Autodesk Inventor part; units mm, degrees
ref_plane "YZ Plane" through (0, 0, 0) normal (1, 0, 0) x (0, 1, 0)
ref_plane "XZ Plane" through (0, 0, 0) normal (0, 1, 0) x (-1, 0, 0)
ref_plane "XY Plane" through (0, 0, 0) normal (0, 0, 1) x (1, 0, 0)
sketch "スケッチ1" plane through (0, 0, 0) normal (0, 0, 1) x (1, 0, 0)
  circle A0 centre (0, 0) radius 1.5
  dimension "d0" = 3
extrude "押し出し1" add sketch "スケッチ1" along normal blind 15
sketch "スケッチ2" plane through (0, 0, 15) normal (0, 0, 1) x (1, 0, 0)
  circle A0 centre (0, 0) radius 1.5
  circle A1 centre (0, 0) radius 3
  dimension "d3" = 6
extrude "押し出し2" add sketch "スケッチ2" along normal blind 2 contours A0 | A1
fillet "フィレット1" radius 2 1 edges at (-3, 0, 17)
properties part number "M3ボタンボルト15" material "鋼、高強度、低合金"
Can you work these out from the model? Positions are in its coordinate system, mm. A direction names the side the tool comes from. Give positions to 0.01 mm unless a question says otherwise; leave off trailing zeros. Loops run counter-clockwise (first coordinate to the right, second up) from the corner with the lowest first, then second, coordinate; pieces in that order, holes last. Notation, with made-up numbers: (28, 62.25) -> (37, 62.25) arc R24 cw to (37, 94.25) -> close; hole circle Ø8 at (-8.75, 11.5). An arc over 180 degrees is marked (long way). Use one line per item in the form item = value.
1) Will these pins go through, and if not, where does the flat tip stop? pin 1 (2 mm diameter, centred on x = 0, z = 12, fed in from -Y); pin 2 (3 mm diameter, centred on x = 2.5, z = 15, fed in from +Y); pin 3 (2 mm diameter, centred on x = -2.5, y = 2, fed in from +Z).
Answers:
pin_1 = -1.5
pin_2 = 2.83
pin_3 = 16.6
2) For faces 1 (the face through (0, 0, 0)), 2 (the face through (-1.5, -0.07, 7.4)), which set-ups out of +Z, -Z, +X, -X, +Y, -Y let a thin tool reach every point of the face, with its end or its side?
Answers:
face_1 = -Z, +X, -X, +Y, -Y
face_2 = -Z
3) If we section it at A-A (z = 13.75): Please give me the cut outline in (x, y).
Answers:
outline = circle Ø3 at (0, 0)
4) I need wall thicknesses on line 1 along Y through (x, z) = (0, 8); line 2 along Z through (x, y) = (-2, -1.5); line 3 along Z through (x, y) = (0.5, -1.25). Which ranges of each line are inside material? Lowest first, please.
Answers:
line_1 = -1.5 to 1.5
line_2 = 15 to 16.32
line_3 = 0 to 16.97
